```python
from build123d import *

# Parameters (mm, degrees)
SKETCH2_W           = 10.5
SKETCH2_H           = 9
BOSS_EXTRUDE2_DEPTH = 1
SKETCH2_3_W         = 11.5
SKETCH2_3_H         = 10
SKETCH2_3_W_2       = 10.5
SKETCH2_3_H_2       = 9
BOSS_EXTRUDE3_DEPTH = 4
SKETCH3_R           = 0.6
CUT_EXTRUDE1_DEPTH  = 10


with BuildPart() as part:
    # Sketch2 → Boss-Extrude2 (new body)
    with BuildSketch(Plane(origin=(0, 0, 0), x_dir=(1, 0, 0), z_dir=(0, 1, 0))):
        with Locations((5.75, 5)):
            Rectangle(SKETCH2_W, SKETCH2_H)
    extrude(amount=BOSS_EXTRUDE2_DEPTH)

    # Sketch2<3> → Boss-Extrude3 (add)
    with BuildSketch(Plane(origin=(0, 0, 0), x_dir=(1, 0, 0), z_dir=(0, 1, 0))):
        with Locations((5.75, 5)):
            Rectangle(SKETCH2_3_W, SKETCH2_3_H)
        with Locations((5.75, 5)):
            Rectangle(SKETCH2_3_W_2, SKETCH2_3_H_2, mode=Mode.SUBTRACT)
    extrude(amount=BOSS_EXTRUDE3_DEPTH)

    # Sketch3 → Cut-Extrude1 (cut)
    with BuildSketch(Plane(origin=(0, 1, 0), x_dir=(1, 0, 0), z_dir=(0, 1, 0))):
        with Locations((5.75, 5)):
            Circle(SKETCH3_R)
    extrude(amount=-CUT_EXTRUDE1_DEPTH, mode=Mode.SUBTRACT)


solid = part.part
```
Part model, mm, in its own coordinate system. A direction names the side the tool comes from. Round coordinates to 2 decimals unless told otherwise and drop trailing zeros. Loops run counter-clockwise (first coordinate to the right, second up) from the corner with the lowest first, then second, coordinate; pieces in that order, holes last. Notation, with made-up numbers: (29.5, 65) -> (86.5, 65) arc R22 ccw to (86.5, 83) -> close; hole circle Ø2 at (15, 64.25). An arc over 180 degrees is marked (long way). Use one line per item in the form item = value. Start each with the question number.
Item 1: Two-plate mould, pull along X, no slides. Class faces 3 (the flat face through (6, 2, -9.5)), 4 (the flat face through (0, 2, -5)), 5 (the flat face through (6, 2, -0.5)), 6 (the flat face through (6, 0, -4)): released by +X, released by -X, zero draft, split by the parting line, or undercut.
Item 2: Band-saw the part on D-D (z = -2). List the corners of the cut face in (x, y).
Item 3: Band-saw the part on A-A (y = 1.4). List the corners of the cut face in (x, z), plus the area to 3 significant figures.
Item 4: Drop flat-ended pins along their axis: pin 1 Ø2.5 at (x, z) = (6, -7) entering from +Y; pin 2 Ø2 at (x, y) = (1.5, 1.5) entering from +Z. Give the stop position or say it passes through.
Item 5: Tool access for faces 1 (the flat face through (6, 2, -10)), 2 (the flat face through (0.5, 2, -5)): list every direction of +Z, -Z, +X, -X, +Y, -Y with a clear straight run to the whole face (end or side of a thin tool).
Item 6: Drill centre lines: line 1 along X through (y, z) = (0.7, -5); line 2 along Z through (x, y) = (5.75, 0.3); line 3 along X through (y, z) = (3.7, -5.5). Where is each one in solid material? Low to high.
Item 7: Band-saw the part on B-B (x = 5.75). List the corners of the cut face in (y, z), plus the area to 3 significant figures.
Item 8: Band-saw the part on C-C (z = -5). List the corners of the cut face in (x, y), plus the area to 3 significant figures.
Data:
q1.face_3 = undercut
q1.face_4 = released by -X
q1.face_5 = undercut
q1.face_6 = zero draft
q2.outline = (0, 0) -> (11.5, 0) -> (11.5, 4) -> (11, 4) -> (11, 1) -> (0.5, 1) -> (0.5, 4) -> (0, 4) -> close
q3.outline = (0, -10) -> (11.5, -10) -> (11.5, 0) -> (0, 0) -> close; hole (0.5, -9.5) -> (11, -9.5) -> (11, -0.5) -> (0.5, -0.5) -> close
q3.area = 20.5 mm^2
q4.pin_1 = 1
q4.pin_2 = 0
q5.face_1 = -Z, +X, -X, +Y, -Y
q5.face_2 = +Y
q6.line_1 = 0 to 5.15, 6.35 to 11.5
q6.line_2 = -10 to -5.6, -4.4 to 0
q6.line_3 = 0 to 0.5, 11 to 11.5
q7.outline = (0, -10) -> (4, -10) -> (4, -9.5) -> (1, -9.5) -> (1, -5.6) -> (0, -5.6) -> close; (0, -4.4) -> (1, -4.4) -> (1, -0.5) -> (4, -0.5) -> (4, 0) -> (0, 0) -> close
q7.area = 11.8 mm^2
q8.outline = (0, 0) -> (5.15, 0) -> (5.15, 1) -> (0.5, 1) -> (0.5, 4) -> (0, 4) -> close; (6.35, 0) -> (11.5, 0) -> (11.5, 4) -> (11, 4) -> (11, 1) -> (6.35, 1) -> close
q8.area = 13.3 mm^2
